Source: CAD feature listing. Evaluate the final solid. Frame: model axes, mm. A direction names the side the tool comes from. Round coordinates to 2 decimals unless told otherwise and drop trailing zeros. Loops run counter-clockwise (first coordinate to the right, second up) from the corner with the lowest first, then second, coordinate; pieces in that order, holes last.
(1) Section B-B, the plane z = 0. Return the cut outline in (x, y), plus the area to 3 significant figures.
(2) First-contact query: pin 1 Ø3 at (x, z) = (-0.5, 21.5) entering from +Y; pin 2 Ø3 at (y, z) = (5, -23.5) entering from -X; pin 3 Ø5 at (x, y) = (-20, 9) entering from -Z. Flat tips, straight axial feed; report the tip coordinate or a pass-through.
(3) Material intervals for probe 1 along X at (y, z) = (4.75, 0); probe 2 along Z at (x, y) = (-15.5, -0.25), sorted ascending.
(4) Set-up query: faces 1 (the cylindrical face through (-2.89, -0.85, 3.77)), 2 (the flat face through (7, 0, 0)). Return all of +Z, -Z, +X, -X, +Y, -Y with unobstructed straight access to the full face (end or side cutting, diameter ignored); none if empty.
(5) Section D-D, the plane x = -18.5. Count the separate pieces of the cut face and the enclosed holes in it, plus the area to 3 significant figures.
(6) Section C-C, the plane y = 5.5. Return the cut outline in (x, z).
(7) Mould query, pull axis Z, two halves, no side actions, for faces 3 (the flat face through (5.2, 0, 33.1)), 4 (the cylindrical face through (17.87, 5.97, -28.04)), 5 (the cylindrical face through (-6.56, 5.97, 29.53)). Classes: pulls with the +Z half, pulls with the -Z half, needs draft (parallel to the pull), parting line crosses it, or undercut.
(8) Section A-A, the plane x = 0. Return the cut outline in (y, z).
```python
from build123d import *

# Parameters (mm, degrees)
SKETCH1_R           = 33.25
SKETCH1_R_2         = 30.25
EXTRUDE_THIN5_DEPTH = 12.1
SKETCH2_R           = 34.25
BOSS_EXTRUDE1_DEPTH = 1.67
SKETCH3_R           = 4.75
CUT_EXTRUDE1_DEPTH  = 2
SKETCH6_R           = 10
CUT_EXTRUDE4_DEPTH  = 2
FILLET1_R           = 2
FILLET2_R           = 2
SKETCH13_R          = 1.75
CUT_EXTRUDE6_DEPTH  = 5


# Read off the part's stored shape, not the designer's step: CSK for M4 Countersunk Flat Head Screw1
with BuildPart() as part:
    # Sketch1 → Extrude-Thin5 (new body)
    with BuildSketch(Plane(origin=(0, 0, 0), x_dir=(1, 0, 0), z_dir=(0, 1, 0))):
        Circle(SKETCH1_R)
        Circle(SKETCH1_R_2, mode=Mode.SUBTRACT)
    extrude(amount=EXTRUDE_THIN5_DEPTH)

    # Sketch2 → Boss-Extrude1 (add)
    with BuildSketch(Plane.XZ):
        with Locations(Location((0, 0, 0), (0, 0, 270))):
            Circle(SKETCH2_R)
    extrude(amount=BOSS_EXTRUDE1_DEPTH)

    # Sketch3 → Cut-Extrude1 (cut)
    with BuildSketch(Plane.XZ.offset(1.67)):
        with Locations(Location((0, 0, 0), (0, 0, 270))):
            Circle(SKETCH3_R)
    extrude(amount=-CUT_EXTRUDE1_DEPTH, mode=Mode.SUBTRACT)

    # Sketch6 → Cut-Extrude4 (cut)
    with BuildSketch(Plane.XZ.offset(1.67)):
        with Locations(Location((-15.156619939, -12.99647525, 0), (0, 0, 270))):
            Circle(SKETCH6_R)
    extrude(amount=-CUT_EXTRUDE4_DEPTH, mode=Mode.SUBTRACT)

    # Fillet1
    # the kernel refuses this fillet: 2 mm, written as the material it takes off along each edge
    with BuildSketch(Plane(origin=(0, -1.67, 0), x_dir=(0, 0, -1), z_dir=(-1, 0, 0))) as fillet1_piece_1:
        with BuildLine():
            CenterArc((32.277412866, -2), FILLET1_R, 9.497234469, 80.502765531)
            Line((32.277412866, 0), (32.277412866, 0.04))
            Line((32.277412866, 0.04), (34.25, 0.04))
            Line((34.25, 0.04), (34.29, 0))
            ThreePointArc((34.29, 0), (34.29, -0.835), (34.289451743, -1.6634))
            Line((34.289451743, -1.6634), (34.25, -1.67))
        make_face()
    revolve(axis=Axis((0, -1.67, 0), (0, -1, 0)), mode=Mode.SUBTRACT)

    # Fillet2
    # the kernel refuses this fillet: 2 mm, written as the material it takes off along each edge
    with BuildSketch(Plane(origin=(-15.156619939, -1.67, -12.99647525), x_dir=(0, 0, -1), z_dir=(-1, 0, 0))) as fillet2_piece_1:
        with BuildLine():
            CenterArc((11.972587134, -2), FILLET2_R, 90, 80.502765531)
            Line((10, -1.67), (9.960548257, -1.6634))
            ThreePointArc((9.960548257, -1.6634), (9.96, -0.835), (9.96, 0))
            Line((9.96, 0), (10, 0.04))
            Line((10, 0.04), (11.972587134, 0.04))
            Line((11.972587134, 0.04), (11.972587134, 0))
        make_face()
    revolve(axis=Axis((-15.156619939, -1.67, -12.99647525), (0, -1, 0)), mode=Mode.SUBTRACT)

    # Sketch13 → Cut-Extrude6 (cut)
    with BuildSketch(Plane.XZ.offset(1.67)):
        with Locations(Location((-16.950332705, 8.520084869, 0), (0, 0, 270))):
            Circle(SKETCH13_R)
        with Locations(Location((17.965530419, 6.094697839, 0), (0, 0, 270))):
            Circle(SKETCH13_R)
    extrude(amount=-CUT_EXTRUDE6_DEPTH, mode=Mode.SUBTRACT)

    # CSK for M4 Countersunk Flat Head Scr 2 → CSK for M4 Countersunk Flat Head Screw1 (revolve, cut)
    with BuildSketch(Plane(origin=(17.965530419, 0, 6.094697839), x_dir=(1, 0, 0), z_dir=(0, 0, 1))):
        Polygon((4.7, 0), (1.75, 0), (1.75, -1.67), (3.03, -1.67), align=None)
    revolve(axis=Axis((17.965530419, 0, 6.094697839), (0, 1, 0)), mode=Mode.SUBTRACT)

    # CSK for M4 Countersunk Flat Head Scr 3 o → CSK for M4 Countersunk Flat Head Scr 3 (revolve, cut)
    with BuildSketch(Plane(origin=(-16.950332705, 0, 8.520084869), x_dir=(1, 0, 0), z_dir=(0, 0, 1))):
        Polygon((4.7, 0), (1.75, 0), (1.75, -1.67), (3.03, -1.67), align=None)
    revolve(axis=Axis((-16.950332705, 0, 8.520084869), (0, 1, 0)), mode=Mode.SUBTRACT)


solid = part.part
```
Output values:
1. outline: (-34.25, 0) arc R2 ccw to (-32.28, -1.67) - (-4.75, -1.67) - (-4.75, 0) - (-30.25, 0) - (-30.25, 12.1) - (-33.25, 12.1) - (-33.25, 0) - close; (4.75, -1.67) - (32.28, -1.67) arc R2 ccw to (34.25, 0) - (33.25, 0) - (33.25, 12.1) - (30.25, 12.1) - (30.25, 0) - (4.75, 0) - close
1. area: 170 mm2
2. pin 1: stops at y = 0
2. pin 2: stops at x = -24.93
2. pin 3: stops at z = -28.27
3. probe 1: x = -33.25 to -30.25, 30.25 to 33.25
3. probe 2: z = -30.48 to -23.05, -2.94 to 4.31, 12.73 to 30.48
4. face 1: +Y, -Y
4. face 2: +Y
5. separate pieces: 3
5. enclosed holes: 0
5. area: 139 mm2
6. outline: circle Ø66.5 at (0, 0); hole circle Ø60.5 at (0, 0)
7. face 3: needs draft
7. face 4: parting line crosses it
7. face 5: undercut
8. outline: (-1.67, -32.28) arc R2 ccw to (0, -34.25) - (0, -33.25) - (12.1, -33.25) - (12.1, -30.25) - (0, -30.25) - (0, -4.75) - (-1.67, -4.75) - close; (-1.67, 4.75) - (0, 4.75) - (0, 30.25) - (12.1, 30.25) - (12.1, 33.25) - (0, 33.25) - (0, 34.25) arc R2 ccw to (-1.67, 32.28) - close
